Autodesk Fusion 360 part; units mm, degrees
sketch "Sketch1" plane through (0, 0, 0) normal (0, 1, 0) x (1, 0, 0)
  line L0 (0, 0) -> (304.8, 0) construction
  line L1 (304.8, 0) -> (304.8, -152.4) construction
  line L2 (304.8, -152.4) -> (0, -152.4) construction
  line L3 (0, -152.4) -> (0, 0) construction
  line L4 (297.775, 0) -> (297.775, -147.9) construction
  line L5 (297.775, -147.9) -> (7.025, -147.9) construction
  line L6 (7.025, -147.9) -> (7.025, 0) construction
  line L7 (39.025, -70.5) -> (76.025, -70.5)
  line L8 (76.025, -70.5) -> (76.025, -132.9)
  line L9 (76.025, -132.9) -> (39.025, -132.9)
  line L10 (39.025, -132.9) -> (39.025, -70.5)
  circle A0 centre (42.95, -74.425) radius 1.625
  line L11 (57.525, -70.5) -> (57.525, -132.9) construction
  circle A1 centre (72.1, -74.425) radius 1.625
  line L12 (39.025, -101.7) -> (76.025, -101.7) construction
  circle A2 centre (72.1, -128.975) radius 1.625
  circle A3 centre (42.95, -128.975) radius 1.625
  line L13 (15.525, -66.5) -> (35.875, -66.5)
  line L14 (35.875, -66.5) -> (35.875, -109.9)
  line L15 (35.875, -109.9) -> (15.525, -109.9)
  line L16 (15.525, -109.9) -> (15.525, -66.5)
  circle A4 centre (18.08, -107.345) radius 1.555
  line L17 (25.7, -66.5) -> (25.7, -109.9) construction
  circle A5 centre (33.32, -107.345) radius 1.555
  line L18 (80.025, -79.56) -> (181.625, -79.56)
  line L19 (181.625, -79.56) -> (181.625, -132.9)
  line L20 (181.625, -132.9) -> (80.025, -132.9)
  line L21 (80.025, -132.9) -> (80.025, -79.56)
  circle A6 centre (85.105, -82.1) radius 1.65
  circle A7 centre (91.455, -130.36) radius 1.65
  circle A8 centre (167.655, -82.1) radius 1.65
  circle A9 centre (166.385, -130.36) radius 1.65
  line L22 (7.025, -52.9) -> (297.775, -52.9) construction
  line L23 (187.625, -82) -> (207.975, -82)
  line L24 (207.975, -82) -> (207.975, -125.4)
  line L25 (207.975, -125.4) -> (187.625, -125.4)
  line L26 (187.625, -125.4) -> (187.625, -82)
  circle A10 centre (190.18, -122.845) radius 1.555
  line L27 (197.8, -82) -> (197.8, -125.4) construction
  circle A11 centre (205.42, -122.845) radius 1.555
  circle A12 centre (145.82, -124.545) radius 1.555
  circle A13 centre (130.58, -124.545) radius 1.555
  line L28 (148.375, -83.7) -> (148.375, -127.1)
  line L29 (148.375, -127.1) -> (128.025, -127.1)
  line L30 (128.025, -127.1) -> (128.025, -83.7)
  line L31 (138.2, -83.7) -> (138.2, -127.1) construction
  line L32 (128.025, -83.7) -> (148.375, -83.7)
  line L33 (215.125, -84.4) -> (281.275, -84.4)
  line L34 (281.275, -84.4) -> (281.275, -120.4)
  line L35 (281.275, -120.4) -> (215.125, -120.4)
  line L36 (215.125, -120.4) -> (215.125, -84.4)
  circle A14 centre (217.675, -86.95) radius 1.55
  line L37 (248.2, -84.4) -> (248.2, -120.4) construction
  line L38 (215.125, -102.4) -> (281.275, -102.4) construction
  circle A15 centre (278.725, -86.95) radius 1.55
  circle A16 centre (217.675, -117.85) radius 1.55
  circle A17 centre (278.725, -117.85) radius 1.55
  line L39 (84.065, -55.86) -> (180.125, -55.86)
  line L40 (180.125, -55.86) -> (180.125, -74.96)
  line L41 (180.125, -74.96) -> (84.065, -74.96)
  line L42 (84.065, -74.96) -> (84.065, -55.86)
  circle A18 centre (177.625, -65.46) radius 1.5
  line L43 (132.095, -55.86) -> (132.095, -74.96) construction
  circle A19 centre (86.565, -65.46) radius 1.5
  line L44 (191.715, -76.4) -> (191.715, -57.3)
  line L45 (239.745, -57.3) -> (239.745, -76.4) construction
  line L46 (287.775, -76.4) -> (191.715, -76.4)
  line L47 (191.715, -57.3) -> (287.775, -57.3)
  circle A20 centre (285.275, -66.9) radius 1.5
  circle A21 centre (194.215, -66.9) radius 1.5
  line L48 (287.775, -57.3) -> (287.775, -76.4)
  line L49 (7.025, -125.9) -> (14.025, -125.9)
  line L50 (14.025, -125.9) -> (14.025, -132.9)
  line L51 (14.025, -132.9) -> (7.025, -132.9)
  line L52 (7.025, -132.9) -> (7.025, -125.9)
  line L53 (7.025, -70.9) -> (14.025, -70.9)
  line L54 (14.025, -70.9) -> (14.025, -77.9)
  line L55 (14.025, -77.9) -> (7.025, -77.9)
  line L56 (7.025, -77.9) -> (7.025, -70.9)
  line L57 (7.025, -39.4) -> (14.025, -39.4)
  line L58 (14.025, -39.4) -> (14.025, -46.4)
  line L59 (14.025, -46.4) -> (7.025, -46.4)
  line L60 (7.025, -46.4) -> (7.025, -39.4)
  line L61 (122.025, -39.4) -> (129.025, -39.4)
  line L62 (129.025, -39.4) -> (129.025, -46.4)
  line L63 (129.025, -46.4) -> (122.025, -46.4)
  line L64 (122.025, -46.4) -> (122.025, -39.4)
  line L65 (152.4, 0) -> (152.4, -147.9) construction
  circle A22 centre (68.025, -8) radius 1.5
  circle A23 centre (10.525, -42.9) radius 1.5
  circle A24 centre (10.525, -74.4) radius 1.5
  circle A25 centre (10.525, -129.4) radius 1.5
  circle A26 centre (125.525, -42.9) radius 1.5
  line L66 (0, 0) -> (304.8, 0)
  line L67 (304.8, 0) -> (304.8, -152.4)
  line L68 (304.8, -152.4) -> (0, -152.4)
  line L69 (0, -152.4) -> (0, 0)
  line L70 (152.4, 0) -> (152.4, -152.4)
  line L71 (-0.1, 0) -> (-2.5, 0)
  line L72 (307.3, 0) -> (304.9, 0)
  line L73 (0, 0) -> (-0.1, 0)
  line L74 (304.9, 0) -> (304.8, 0)
  line L75 (184.625, 0) -> (184.625, -152.4)
  line L76 (165, 0) -> (165, -50)
  line L77 (165, -50) -> (184.625, -50)
  circle A27 centre (24, -128.4) radius 3.95
  line L78 (0, -76.2) -> (304.8, -76.2) construction
  circle A28 centre (24, -24) radius 3.95
  circle A29 centre (280.8, -24) radius 3.95
  circle A30 centre (280.8, -128.4) radius 3.95
  circle A31 centre (147.4, -4.75) radius 1.5
  circle A32 centre (157.4, -4.75) radius 1.5
  line L79 (64.525, -4.5) -> (71.525, -4.5)
  line L80 (71.525, -4.5) -> (71.525, -11.5)
  line L81 (71.525, -11.5) -> (64.525, -11.5)
  line L82 (64.525, -11.5) -> (64.525, -4.5)
  line L83 (233.275, -11.5) -> (240.275, -11.5)
  circle A33 centre (236.775, -8) radius 1.5
  line L84 (240.275, -11.5) -> (240.275, -4.5)
  line L85 (240.275, -4.5) -> (233.275, -4.5)
  line L86 (233.275, -4.5) -> (233.275, -11.5)
  line L87 (297.775, -39.4) -> (290.775, -39.4)
  line L88 (290.775, -39.4) -> (290.775, -46.4)
  circle A34 centre (294.275, -42.9) radius 1.5
  line L89 (290.775, -46.4) -> (297.775, -46.4)
  line L90 (297.775, -46.4) -> (297.775, -39.4)
  line L91 (297.775, -70.9) -> (290.775, -70.9)
  line L92 (290.775, -70.9) -> (290.775, -77.9)
  circle A35 centre (294.275, -74.4) radius 1.5
  line L93 (297.775, -77.9) -> (297.775, -70.9)
  line L94 (290.775, -77.9) -> (297.775, -77.9)
  line L95 (297.775, -125.9) -> (290.775, -125.9)
  line L96 (290.775, -125.9) -> (290.775, -132.9)
  circle A36 centre (294.275, -129.4) radius 1.5
  line L97 (290.775, -132.9) -> (297.775, -132.9)
  line L98 (297.775, -132.9) -> (297.775, -125.9)
  circle A37 centre (179.275, -42.9) radius 1.5
  line L99 (175.775, -46.4) -> (182.775, -46.4)
  line L100 (182.775, -46.4) -> (182.775, -39.4)
  line L101 (175.775, -39.4) -> (175.775, -46.4)
  line L102 (182.775, -39.4) -> (175.775, -39.4)
  dimension "d1" = 304.8
  dimension "d2" = 152.4
  dimension "d3" = 290.75
  dimension "d4" = 147.9
  dimension "d5" = 7.025
  dimension "d6" = 3.25
  dimension "d7" = 37
  dimension "d8" = 62.4
  dimension "d9" = 3.925
  dimension "d10" = 3.925
  dimension "d11" = 32
  dimension "d13" = 20.35
  dimension "d14" = 43.4
  dimension "d15" = 3.11
  dimension "d16" = 2.555
  dimension "d17" = 2.555
  dimension "d18" = 8.5
  dimension "d19" = 42.5
  dimension "d20" = 19.5
  dimension "d21" = 101.6
  dimension "d22" = 53.34
  dimension "d23" = 3.3
  dimension "d24" = 3.3
  dimension "d25" = 3.3
  dimension "d26" = 3.3
  dimension "d27" = 96.52
  dimension "d28" = 2.54
  dimension "d29" = 13.97
  dimension "d30" = 2.54
  dimension "d31" = 15.24
  dimension "d32" = 50.8
  dimension "d33" = 90.17
  dimension "d34" = 50.8
  dimension "d35" = 19.5
  dimension "d36" = 73
  dimension "d38" = 20.35
  dimension "d39" = 43.4
  dimension "d40" = 3.11
  dimension "d41" = 2.555
  dimension "d42" = 2.555
  dimension "d43" = 27
  dimension "d45" = 6
  dimension "d46" = 20.35
  dimension "d47" = 43.4
  dimension "d48" = 3.11
  dimension "d49" = 2.555
  dimension "d50" = 2.555
  dimension "d51" = 25.3
  dimension "d52" = 48
  dimension "d53" = 66.15
  dimension "d54" = 36
  dimension "d55" = 3.1
  dimension "d56" = 2.55
  dimension "d57" = 2.55
  dimension "d58" = 32
  dimension "d59" = 16.5
  dimension "d60" = 96.06
  dimension "d61" = 19.1
  dimension "d62" = 3
  dimension "d63" = 9.6
  dimension "d64" = 2.5
  dimension "d65" = 4.6
  dimension "d66" = 1.5
  dimension "d67" = 96.06
  dimension "d68" = 19.1
  dimension "d69" = 3
  dimension "d70" = 9.6
  dimension "d71" = 2.5
  dimension "d72" = 10
  dimension "d73" = 8
  dimension "d74" = 7
  dimension "d75" = 7
  dimension "d76" = 15
  dimension "d77" = 7
  dimension "d78" = 7
  dimension "d79" = 70
  dimension "d80" = 7
  dimension "d81" = 7
  dimension "d82" = 101.5
  dimension "d86" = 7
  dimension "d87" = 7
  dimension "d88" = 115
  dimension "d89" = 101.5
  dimension "d90" = 3
  dimension "d93" = 3
  dimension "d94" = 3.5
  dimension "d95" = 3.5
  dimension "d96" = 3
  dimension "d97" = 3.5
  dimension "d98" = 3.5
  dimension "d99" = 3
  dimension "d100" = 3.5
  dimension "d101" = 3.5
  dimension "d102" = 3
  dimension "d103" = 3.5
  dimension "d104" = 3.5
  dimension "d127" = 3
  dimension "d130" = 19.625
  dimension "d131" = 50
  dimension "d132" = 7.9
  dimension "d133" = 24
  dimension "d134" = 24
  dimension "d135" = 3
  dimension "d136" = 3
  dimension "d137" = 10
  dimension "d140" = 5
  dimension "d141" = 4.75
  dimension "d145" = 7
  dimension "d146" = 7
  dimension "d147" = 3.5
  dimension "d148" = 3.5
  dimension "d149" = 4.5
  dimension "d150" = 4.75
  dimension "d151" = 57.5
  dimension "d152" = 52.9
extrude "Extrude7" add sketch "Sketch1" along normal blind 1 contours L7 L8 L9 L10 | L13 L14 L15 L16 | L18 L20 L21 L39 L41 L42 L66 L68 L69 L70 | L18 L20 L21 L70 | L18 L19 L20 L39 L40 L41 L66 L68 L70 L75 L76 L77 | L18 L19 L20 L70 | L39 L40 L41 L70 | L39 L41 L42 L70 | L28 L29 L30 L32 | L49 L50 L51 L52 | L53 L54 L55 L56 | L57 L58 L59 L60 | L61 L62 L63 L64 | L79 L80 L81 L82
equation "d3 = 297.75 mm - ( 3.5 * 2 ) * 1 mm"
equation "d5 = ( d1 - d3 ) / 2"
equation "d9 = d6 / 2 + 2.3 mm"
equation "d10 = d9"
equation "d16 = d15 / 2 + 1 mm"
equation "d17 = d16"
equation "d24 = d23"
equation "d25 = d23"
equation "d26 = d23"
equation "d30 = d28"
equation "d34 = d32"
equation "d41 = d15 / 2 + 1 mm"
equation "d42 = d16"
equation "d49 = d15 / 2 + 1 mm"
equation "d50 = d16"
equation "d56 = d55 / 2 + 1 mm"
equation "d57 = d55 / 2 + 1 mm"
equation "d63 = d62 / 2 + 8.1 mm"
equation "d64 = d62 / 2 + 1 mm"
equation "d70 = d62 / 2 + 8.1 mm"
equation "d71 = d62 / 2 + 1 mm"
equation "d94 = d80 / 2"
equation "d95 = d81 / 2"
equation "d97 = d78 / 2"
equation "d98 = d77 / 2"
equation "d100 = d74 / 2"
equation "d101 = d75 / 2"
equation "d103 = d87 / 2"
equation "d104 = d86 / 2"
equation "d140 = d137 / 2"
equation "d147 = d145 / 2"
equation "d148 = d146 / 2"
The listing builds one solid part. Answer for the finished solid, in the listing's coordinates (mm). Coordinates: 2 decimals unless noted, no trailing zeros. Write each loop counter-clockwise with the first axis right and the second up, starting at its lowest first coordinate (ties: lowest second). Pieces come first, ordered by that corner, then holes. Notation, with made-up numbers: M 29,25.25 L 42,25.25 A10 ccw 42,44.25 Z; hole C 79,77 d6. An arc over 180 degrees is marked long. Use a Markdown table: item, result. Add a question column.
1. Straight lines are drawn through the part: line 1 along Z through (x, y) = (42.95, 0.75); line 2 along Z through (x, y) = (157.4, 0.6); line 3 along Z through (x, y) = (24, 0.6). For each, find the intervals that lie inside material, in ascending order. Write a range as [from, to].
2. Section C-C (z = 47) is taken. Give the vertices of the cut face in (x, y).
3. Given P1, Ø1.9, axis at x = 42.95, z = 128.975, coming from the +Y side; P2, Ø0.5, axis at x = 175.5, y = 0.5, coming from the -Z side, each flat-ended and moving along its own axis, determine where each tip first touches the part or whether it passes through.
4. Section B-B (z = 24) is taken. Give the vertices of the cut face in (x, y).
5. Section A-A (x = 24) is taken. Give the vertices of the cut face in (y, z).
6. For a pull along X with two mould halves and no side action, classify faces 1 (the cylindrical face through (23.144, 0.493, 124.544)), 2 (the flat face through (91, 0, 75)) as +X half, -X half, draft (parallel to the pull), parting line (faces both ways), or undercut.
Data:
| question | item | result |
|---|---|---|
| 1 | line 1 | z = [0, 72.8], [76.05, 127.35], [130.6, 152.4] |
| 1 | line 2 | z = [0, 3.25], [6.25, 152.4] |
| 1 | line 3 | z = [0, 20.05], [27.95, 124.45], [132.35, 152.4] |
| 2 | outline | M 0,0 L 165,0 L 165,1 L 0,1 Z |
| 3 | P1 | passes through |
| 3 | P2 | stops at z = 50 |
| 4 | outline | M 0,0 L 20.05,0 L 20.05,1 L 0,1 Z; M 27.95,0 L 165,0 L 165,1 L 27.95,1 Z |
| 5 | outline | M 0,0 L 1,0 L 1,20.05 L 0,20.05 Z; M 0,27.95 L 1,27.95 L 1,124.45 L 0,124.45 Z; M 0,132.35 L 1,132.35 L 1,152.4 L 0,152.4 Z |
| 6 | face 1 | undercut |
| 6 | face 2 | draft |
